Can you work these out from the model? Positions are in its coordinate system, mm. Face numbers are marked on the shaded views. Round coordinates to 2 decimals unless told otherwise and drop trailing zeros. Order: outer loops, then holes, each group sorted by start corner. A loop starts at its lowest first (then second) coordinate and runs counter-clockwise, first axis right, second up. Notation, with made-up numbers: (4.25, -3.5) - (42.25, -3.5) arc R19 ccw to (42.25, 9.5) - close; hole circle Ø11 at (62.5, 87.5). An arc over 180 degrees is marked (long way). Write item = value, one per line.
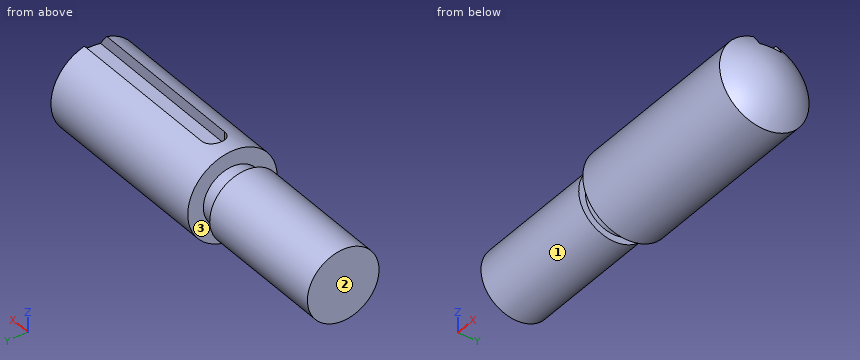
from build123d import *

# Parameters (mm, degrees)
ENL_V_MAT_EXTRU_1_DEPTH = 3


with BuildPart() as part:
    # Esquisse1 → Révolution1 (revolve)
    with BuildSketch(Plane.XY, mode=Mode.PRIVATE) as r_volution1_sk:
        with BuildLine():
            Line((80, 0), (0, 0))
            Line((0, 0), (0, 8))
            Line((0, 8), (30, 8))
            Line((30, 8), (30, 6.5))
            Line((30, 6.5), (34, 6.5))
            Line((34, 6.5), (34, 10))
            Line((34, 10), (76, 10))
            ThreePointArc((76, 10), (78.962912018, 5.385164807), (80, 0))
        make_face()
    revolve(r_volution1_sk.sketch.rotate(Axis((80, 0, 0), (-1, 0, 0)), 90), axis=Axis((80, 0, 0), (-1, 0, 0)))

    # Esquisse2 → Enlèv. mat.-Extru.1 (cut)
    with BuildSketch(Plane.XY.offset(10)):
        with BuildLine():
            Line((39.924742885, 2.51802815), (89.396583104, 2.51802815))
            Line((89.396583104, 2.51802815), (89.396583104, -2.514235284))
            Line((89.396583104, -2.514235284), (39.924742885, -2.514235284))
            ThreePointArc((39.924742885, -2.514235284), (37.408611168, 0.001896433), (39.924742885, 2.51802815))
        make_face()
    extrude(amount=-ENL_V_MAT_EXTRU_1_DEPTH, mode=Mode.SUBTRACT)


solid = part.part
(1) Will these pins go through, and if not, where does the flat tip stop? P1, Ø0.8, axis at x = 68, z = 8, coming from the +Y side; P2, Ø10, axis at y = -5, z = -3.5, coming from the +X side; P3, Ø8, axis at x = 27.5, z = -6, coming from the -Y side.
Computed:
P1 = 6.5
P2 = 79.96
P3 = -7.75
(2) If we section it at B-B (y = 0): Write out the boundary of the cut face in (x, z), plus the area to 3 significant figures.
Computed:
outline = (0, -8) - (30, -8) - (30, -6.5) - (34, -6.5) - (34, -10) - (76, -10) arc R14.5 ccw to (78.2, 7) - (37.41, 7) - (37.41, 10) - (34, 10) - (34, 6.5) - (30, 6.5) - (30, 8) - (0, 8) - close
area = 1,310 mm^2
(3) If we section it at D-D (z = -4.75): Write out the boundary of the cut face in (x, y).
Computed:
outline = (0, -6.44) - (30, -6.44) - (30, -4.44) - (34, -4.44) - (34, -8.8) - (76, -8.8) arc R13.7 ccw to (76, 8.8) - (34, 8.8) - (34, 4.44) - (30, 4.44) - (30, 6.44) - (0, 6.44) - close
(4) If we section it at A-A (z = 0): Write out the boundary of the cut face in (x, y).
Computed:
outline = (0, -8) - (30, -8) - (30, -6.5) - (34, -6.5) - (34, -10) - (76, -10) arc R14.5 ccw to (76, 10) - (34, 10) - (34, 6.5) - (30, 6.5) - (30, 8) - (0, 8) - close
(5) If I drill on line 1 (Y direction, x = 45.5, z = 9); line 2 (X direction, y = 7, z = -3.5); line 3 (Y direction, x = 55.5, z = 7.5), over which ranges is the centre line in solid material (lowest first)? Write a range as from..to.
Computed:
line_1 = -4.36..-2.51, 2.52..4.36
line_2 = 0..30, 34..77.71
line_3 = -6.61..-2.51, 2.52..6.61
(6) If we section it at C-C (x = 43): Write out the boundary of the cut face in (y, z), plus the area to 3 significant figures.
Computed:
outline = (-2.51, 7) - (-2.51, 9.68) arc R10 ccw (long way) to (2.52, 9.68) - (2.52, 7) - close
area = 300 mm^2
(7) Thinking about a two-plate mould opening in X: for the marked faces 1, 2 and 3, which applies, +X half, -X half, draft (parallel to the pull), parting line (faces both ways), or undercut?
Computed:
face_1 = draft
face_2 = -X half
face_3 = undercut
